Autodesk Fusion 360 part; units mm, degrees
sketch "Sketch1" plane through (0, 0, 0) normal (0, 1, 0) x (1, 0, 0)
  line L0 (0, 0) -> (10, 0)
  line L1 (10, 0) -> (10, -27)
  line L2 (10, -27) -> (0, -27)
  line L3 (0, -27) -> (0, 0)
  line L4 (0, -19.5) -> (5, -19.5)
  line L5 (5, -19.5) -> (5, -7.5)
  line L6 (5, -7.5) -> (0, -7.5)
  line L7 (0, -7.5) -> (0, -19.5)
  dimension "d1" = 10
  dimension "d2" = 27
  dimension "d3" = 12
  dimension "d4" = 5
  dimension "d6" = 7.5
extrude "Extrude1" add sketch "Sketch1" along normal blind 34.7 contours L0 L1 L2 L3 L4 L5 L6
sketch "Sketch2" plane through (10, 0, 0) normal (1, 0, 0) x (0, 1, 0)
  line L0 (0, 27) -> (0, 0)
  line L1 (0, 0) -> (34.7, 0)
  line L2 (34.7, 0) -> (34.7, 27)
  line L3 (34.7, 27) -> (0, 27)
  line L4 (7.35, 3.5) -> (27.35, 3.5)
  line L5 (27.35, 3.5) -> (27.35, 23.5)
  line L6 (27.35, 23.5) -> (7.35, 23.5)
  line L7 (7.35, 23.5) -> (7.35, 3.5)
  circle A0 centre (7.35, 23.5) radius 1.5
  circle A1 centre (27.35, 23.5) radius 1.5
  circle A2 centre (7.35, 3.5) radius 1.5
  circle A3 centre (27.35, 3.5) radius 1.5
  dimension "d9" = 20
  dimension "d10" = 20
  dimension "d11" = 3.5
  dimension "d12" = 7.35
  dimension "d13" = 3
  dimension "d14" = 3
  dimension "d15" = 3
  dimension "d16" = 3
extrude "Extrude2" cut sketch "Sketch2" against normal blind 5 contours L4 L7 A2 | L4 L7 A2 | L4 L5 A3 | L4 L5 A3 | L6 L7 A0 | L6 L7 A0 | L5 L6 A1 | L5 L6 A1
equation "d12 = 9.85 mm - 2.5 mm"
The model under review builds one solid part; all positions refer to its coordinate system, in mm. A direction names the side the tool comes from. Give positions to 0.01 mm unless a question says otherwise; leave off trailing zeros. Write each loop counter-clockwise with the first axis right and the second up, starting at its lowest first coordinate (ties: lowest second). Pieces come first, ordered by that corner, then holes. Notation, with made-up numbers: M 50.5,25.5 L 99.5,25.5 A32 ccw 99.5,61.5 Z; hole C 57.5,51.5 d7. An arc over 180 degrees is marked long. Answer in a Markdown table with one row per item.
Item 1: Add section D-D on z = 3.5. Give the boundary of the cut face in (x, y).
Check sheet entries:
| item | result |
|---|---|
| outline | M 0,0 L 10,0 L 10,5.85 L 5,5.85 L 5,8.85 L 10,8.85 L 10,25.85 L 5,25.85 L 5,28.85 L 10,28.85 L 10,34.7 L 0,34.7 Z |
Item 2: Add section A-A on x = 1.75. Give the boundary of the cut face in (y, z), plus the area to 4 significant figures.
Check sheet entries:
| item | result |
|---|---|
| outline | M 0,0 L 34.7,0 L 34.7,7.5 L 0,7.5 Z; M 0,19.5 L 34.7,19.5 L 34.7,27 L 0,27 Z |
| area | 520.5 mm2 |
Item 3: Draft analysis for pull direction Z (two halves, no side actions). For faces 1 (the face through (7.535, 8.736, 2.925)), 2 (the face through (6, 34.7, 13)), 3 (the face through (5, 17, 14)), 4 (the face through (5, 17, 27)), state which applies: +Z half, -Z half, draft (parallel to the pull), parting line (faces both ways), or undercut.
Check sheet entries:
| item | result |
|---|---|
| face 1 | undercut |
| face 2 | draft |
| face 3 | undercut |
| face 4 | +Z half |
Item 4: Add section B-B on y = 7.35. Give the boundary of the cut face in (x, z), plus the area to 3 significant figures.
Check sheet entries:
| item | result |
|---|---|
| outline | M 0,0 L 10,0 L 10,2 L 5,2 L 5,5 L 10,5 L 10,22 L 5,22 L 5,25 L 10,25 L 10,27 L 0,27 L 0,19.5 L 5,19.5 L 5,7.5 L 0,7.5 Z |
| area | 180 mm2 |
Item 5: For line 1 along Y through (x, z) = (7.3, 3.5); line 2 along Z through (x, y) = (7.8, 27.35); line 3 along Z through (x, y) = (4, 26), list the stretches that pass through material, from the lowest coordinate up.
Check sheet entries:
| item | result |
|---|---|
| line 1 | 0 to 5.85, 8.85 to 25.85, 28.85 to 34.7 |
| line 2 | 0 to 2, 5 to 22, 25 to 27 |
| line 3 | 0 to 7.5, 19.5 to 27 |
Item 6: For P1, Ø1.5, axis at y = 7, z = 4, coming from the +X side; P2, Ø1.5, axis at y = 21.5, z = 18.5, coming from the -X side, all flat-tipped, find the tip position at first contact; note any pin that passes through.
Check sheet entries:
| item | result |
|---|---|
| P1 | x = 5 |
| P2 | x = 5 |
Item 7: Tool access review of faces 5 (the face through (3, 17, 7.5)), 6 (the face through (7.54, 25.85, 3.57)), 7 (the face through (5, 17, 0)): name each direction out of +Z, -Z, +X, -X, +Y, -Y from which nothing blocks a thin tool from reaching the whole face with its end or side.
Check sheet entries:
| item | result |
|---|---|
| face 5 | -X, +Y, -Y |
| face 6 | +X |
| face 7 | -Z, +X, -X, +Y, -Y |
Item 8: Add section C-C on x = 6.5. Give the boundary of the cut face in (y, z), plus the area to 3 significant figures.
Check sheet entries:
| item | result |
|---|---|
| outline | M 0,0 L 34.7,0 L 34.7,27 L 0,27 Z; hole C 7.35,3.5 d3; hole C 7.35,23.5 d3; hole C 27.35,3.5 d3; hole C 27.35,23.5 d3 |
| area | 909 mm2 |
